Could you check a few things on this model? Use its own coordinates, in mm. Face numbers are marked on the shaded views. A direction names the side the tool comes from. Coordinates: 2 decimals unless noted, no trailing zeros. Write each loop counter-clockwise with the first axis right and the second up, starting at its lowest first coordinate (ties: lowest second). Pieces come first, ordered by that corner, then holes.
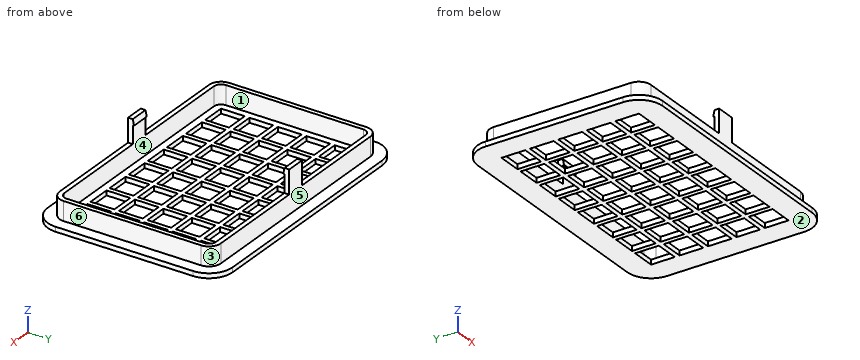
```python
from build123d import *

# Parameters (mm, degrees)
F0_W     = 10
F0_H     = 10
F1_DEPTH = 2
F2_DEPTH = 10
F3_W     = 8
F3_H     = 2
F4_DEPTH = 10
F6_DEPTH = 8


with BuildPart() as f1:
    # F0 (on Top) → F1 (new body)
    with BuildSketch(Plane.XY):
        with BuildLine():
            ThreePointArc((0, 10), (2.9289321881, 2.9289321881), (10, 0))
            Line((10, 0), (104, 0))
            ThreePointArc((104, 0), (111.0710678119, 2.9289321881), (114, 10))
            Line((114, 10), (114, 68))
            ThreePointArc((114, 68), (111.0710678119, 75.0710678119), (104, 78))
            Line((104, 78), (10, 78))
            ThreePointArc((10, 78), (2.9289321881, 75.0710678119), (0, 68))
            Line((0, 68), (0, 10))
        make_face()
        with BuildLine():
            ThreePointArc((10, 5), (6.4644660941, 6.4644660941), (5, 10))
            Line((5, 10), (5, 68))
            ThreePointArc((5, 68), (6.4644660941, 71.5355339059), (10, 73))
            Line((10, 73), (104, 73))
            ThreePointArc((104, 73), (107.5355339059, 71.5355339059), (109, 68))
            Line((109, 68), (109, 10))
            ThreePointArc((109, 10), (107.5355339059, 6.4644660941), (104, 5))
            Line((104, 5), (10, 5))
        make_face(mode=Mode.SUBTRACT)
        with BuildLine():
            Line((5, 68), (5, 10))
            ThreePointArc((5, 10), (6.4644660941, 6.4644660941), (10, 5))
            Line((10, 5), (104, 5))
            ThreePointArc((104, 5), (107.5355339059, 6.4644660941), (109, 10))
            Line((109, 10), (109, 68))
            ThreePointArc((109, 68), (107.5355339059, 71.5355339059), (104, 73))
            Line((104, 73), (10, 73))
            ThreePointArc((10, 73), (6.4644660941, 71.5355339059), (5, 68))
        make_face()
        with BuildLine():
            ThreePointArc((10, 7), (7.8786796564, 7.8786796564), (7, 10))
            Line((7, 10), (7, 68))
            ThreePointArc((7, 68), (7.8786796564, 70.1213203436), (10, 71))
            Line((10, 71), (104, 71))
            ThreePointArc((104, 71), (106.1213203436, 70.1213203436), (107, 68))
            Line((107, 68), (107, 10))
            ThreePointArc((107, 10), (106.1213203436, 7.8786796564), (104, 7))
            Line((104, 7), (10, 7))
        make_face(mode=Mode.SUBTRACT)
        with BuildLine():
            Line((7, 68), (7, 10))
            ThreePointArc((7, 10), (7.8786796564, 7.8786796564), (10, 7))
            Line((10, 7), (104, 7))
            ThreePointArc((104, 7), (106.1213203436, 7.8786796564), (107, 10))
            Line((107, 10), (107, 68))
            ThreePointArc((107, 68), (106.1213203436, 70.1213203436), (104, 71))
            Line((104, 71), (10, 71))
            ThreePointArc((10, 71), (7.8786796564, 70.1213203436), (7, 68))
        make_face()
        with Locations((15, 15)):
            Rectangle(F0_W, F0_H, mode=Mode.SUBTRACT)
        with Locations((27, 15)):
            Rectangle(F0_W, F0_H, mode=Mode.SUBTRACT)
        with Locations((39, 15)):
            Rectangle(F0_W, F0_H, mode=Mode.SUBTRACT)
        with Locations((51, 15)):
            Rectangle(F0_W, F0_H, mode=Mode.SUBTRACT)
        with Locations((15, 27)):
            Rectangle(F0_W, F0_H, mode=Mode.SUBTRACT)
        with Locations((27, 27)):
            Rectangle(F0_W, F0_H, mode=Mode.SUBTRACT)
        with Locations((39, 27)):
            Rectangle(F0_W, F0_H, mode=Mode.SUBTRACT)
        with Locations((51, 27)):
            Rectangle(F0_W, F0_H, mode=Mode.SUBTRACT)
        with Locations((63, 15)):
            Rectangle(F0_W, F0_H, mode=Mode.SUBTRACT)
        with Locations((75, 15)):
            Rectangle(F0_W, F0_H, mode=Mode.SUBTRACT)
        with Locations((87, 15)):
            Rectangle(F0_W, F0_H, mode=Mode.SUBTRACT)
        with Locations((99, 15)):
            Rectangle(F0_W, F0_H, mode=Mode.SUBTRACT)
        with Locations((63, 27)):
            Rectangle(F0_W, F0_H, mode=Mode.SUBTRACT)
        with Locations((75, 27)):
            Rectangle(F0_W, F0_H, mode=Mode.SUBTRACT)
        with Locations((87, 27)):
            Rectangle(F0_W, F0_H, mode=Mode.SUBTRACT)
        with Locations((99, 27)):
            Rectangle(F0_W, F0_H, mode=Mode.SUBTRACT)
        with Locations((15, 39)):
            Rectangle(F0_W, F0_H, mode=Mode.SUBTRACT)
        with Locations((27, 39)):
            Rectangle(F0_W, F0_H, mode=Mode.SUBTRACT)
        with Locations((15, 51)):
            Rectangle(F0_W, F0_H, mode=Mode.SUBTRACT)
        with Locations((27, 51)):
            Rectangle(F0_W, F0_H, mode=Mode.SUBTRACT)
        with Locations((39, 39)):
            Rectangle(F0_W, F0_H, mode=Mode.SUBTRACT)
        with Locations((51, 39)):
            Rectangle(F0_W, F0_H, mode=Mode.SUBTRACT)
        with Locations((39, 51)):
            Rectangle(F0_W, F0_H, mode=Mode.SUBTRACT)
        with Locations((51, 51)):
            Rectangle(F0_W, F0_H, mode=Mode.SUBTRACT)
        with Locations((15, 63)):
            Rectangle(F0_W, F0_H, mode=Mode.SUBTRACT)
        with Locations((27, 63)):
            Rectangle(F0_W, F0_H, mode=Mode.SUBTRACT)
        with Locations((39, 63)):
            Rectangle(F0_W, F0_H, mode=Mode.SUBTRACT)
        with Locations((51, 63)):
            Rectangle(F0_W, F0_H, mode=Mode.SUBTRACT)
        with Locations((63, 39)):
            Rectangle(F0_W, F0_H, mode=Mode.SUBTRACT)
        with Locations((75, 39)):
            Rectangle(F0_W, F0_H, mode=Mode.SUBTRACT)
        with Locations((63, 51)):
            Rectangle(F0_W, F0_H, mode=Mode.SUBTRACT)
        with Locations((75, 51)):
            Rectangle(F0_W, F0_H, mode=Mode.SUBTRACT)
        with Locations((87, 39)):
            Rectangle(F0_W, F0_H, mode=Mode.SUBTRACT)
        with Locations((99, 39)):
            Rectangle(F0_W, F0_H, mode=Mode.SUBTRACT)
        with Locations((87, 51)):
            Rectangle(F0_W, F0_H, mode=Mode.SUBTRACT)
        with Locations((99, 51)):
            Rectangle(F0_W, F0_H, mode=Mode.SUBTRACT)
        with Locations((63, 63)):
            Rectangle(F0_W, F0_H, mode=Mode.SUBTRACT)
        with Locations((75, 63)):
            Rectangle(F0_W, F0_H, mode=Mode.SUBTRACT)
        with Locations((87, 63)):
            Rectangle(F0_W, F0_H, mode=Mode.SUBTRACT)
        with Locations((99, 63)):
            Rectangle(F0_W, F0_H, mode=Mode.SUBTRACT)
    extrude(amount=F1_DEPTH)

    # F0 (on Top) → F2 (join)
    with BuildSketch(Plane.XY):
        with BuildLine():
            Line((5, 68), (5, 10))
            ThreePointArc((5, 10), (6.4644660941, 6.4644660941), (10, 5))
            Line((10, 5), (104, 5))
            ThreePointArc((104, 5), (107.5355339059, 6.4644660941), (109, 10))
            Line((109, 10), (109, 68))
            ThreePointArc((109, 68), (107.5355339059, 71.5355339059), (104, 73))
            Line((104, 73), (10, 73))
            ThreePointArc((10, 73), (6.4644660941, 71.5355339059), (5, 68))
        make_face()
        with BuildLine():
            ThreePointArc((10, 7), (7.8786796564, 7.8786796564), (7, 10))
            Line((7, 10), (7, 68))
            ThreePointArc((7, 68), (7.8786796564, 70.1213203436), (10, 71))
            Line((10, 71), (104, 71))
            ThreePointArc((104, 71), (106.1213203436, 70.1213203436), (107, 68))
            Line((107, 68), (107, 10))
            ThreePointArc((107, 10), (106.1213203436, 7.8786796564), (104, 7))
            Line((104, 7), (10, 7))
        make_face(mode=Mode.SUBTRACT)
    extrude(amount=F2_DEPTH)

    # F3 (on face) → F4 (join)
    with BuildSketch(Plane.XY.offset(10)):
        with Locations((57, 72)):
            Rectangle(F3_W, F3_H)
        with Locations((57, 6)):
            Rectangle(F3_W, F3_H)
    extrude(amount=F4_DEPTH)

    # F5 (on face) → F6 (join, through all)
    with BuildSketch(Plane(origin=(53, 0, 0), x_dir=(0, -1, 0), z_dir=(-1, 0, 0))):
        Polygon((-70.5, 17.5), (-71, 20), (-71, 17.5), align=None)
        Polygon((-7, 20), (-7.5, 17.5), (-7, 17.5), align=None)
    extrude(amount=-F6_DEPTH)


solid = f1.part
```
1. Please list where these lines run through material, in increasing order: line 1 along Y through (x, z) = (58, 4); line 2 along X through (y, z) = (16.5, 3); line 3 along Z through (x, y) = (95, 45.5).
Verdict:
line 1: y = 5 to 7, 71 to 73
line 2: x = 5 to 7, 107 to 109
line 3: z = 0 to 2
2. I want a section at C-C on z = 16.25. Please give me the cut outline in (x, y).
Verdict:
outline: (53, 5) - (61, 5) - (61, 7) - (53, 7) - close; (53, 71) - (61, 71) - (61, 73) - (53, 73) - close
3. On a 3-axis mill with a long thin cutter (end or side, diameter ignored), from which of +Z, -Z, +X, -X, +Y, -Y can I reach the whole of each face in a straight line? I mean the marked faces 1, 2 and 3. Say none if no direction works.
Verdict:
face 1: +Z
face 2: -Z, +X, -X, +Y, -Y
face 3: +Z, +X, +Y
4. I want a section at B-B on z = 7. Please give me the cut outline in (x, y).
Verdict:
outline: (5, 10) arc R5 ccw to (10, 5) - (104, 5) arc R5 ccw to (109, 10) - (109, 68) arc R5 ccw to (104, 73) - (10, 73) arc R5 ccw to (5, 68) - close; hole (7, 10) arc R3 ccw to (10, 7) - (104, 7) arc R3 ccw to (107, 10) - (107, 68) arc R3 ccw to (104, 71) - (10, 71) arc R3 ccw to (7, 68) - close
5. If we mould it in two halves opening along Y, with no side actions, what happens to the marked faces 4, 5 and 6? For each: pulls with the +Y half, pulls with the -Y half, needs draft (parallel to the pull), parting line crosses it, or undercut.
Verdict:
face 4: undercut
face 5: pulls with the +Y half
face 6: needs draft
6. For pin 1 (1 mm diameter, centred on y = 41.5, z = 9, fed in from +X); pin 2 (2 mm diameter, centred on y = 26, z = 0.5, fed in from -X); pin 3 (4 mm diameter, centred on y = 26.5, z = 5, fed in from -X); pin 4 (4 mm diameter, centred on x = 91, y = 69.5, fed in from +Z), each with a flat end and sliding along its axis, tell me the tip position at first contact or that it passes through.
Verdict:
pin 1: stops at x = 109
pin 2: stops at x = 0
pin 3: stops at x = 5
pin 4: stops at z = 10
7. I want a section at A-A on x = 72. Give the number of separate pieces and of enclosed holes in the cut face, plus the area to 3 significant figures.
Verdict:
separate pieces: 6
enclosed holes: 0
area: 88.0 mm2
